```python
from build123d import *

# Parameters (mm, degrees)
SKETCH1_W           = 100
SKETCH1_H           = 40
BOSS_EXTRUDE1_DEPTH = 5
BOSS_EXTRUDE2_DEPTH = 5
SKETCH4_W           = 40
SKETCH4_H           = 12
BOSS_EXTRUDE3_DEPTH = 20
CUT_EXTRUDE2_DEPTH  = 70
BOSS_EXTRUDE5_DEPTH = 100
SKETCH12_R          = 1.4
CUT_EXTRUDE3_DEPTH  = 10
CUT_EXTRUDE4_DEPTH  = 30
BOSS_EXTRUDE6_DEPTH = 25
CUT_EXTRUDE5_DEPTH  = 30
BOSS_EXTRUDE7_DEPTH = 25
FILLET1_R           = 5


with BuildPart() as part:
    # Sketch1 → Boss-Extrude1 (new body)
    with BuildSketch(Plane(origin=(0, 0, 0), x_dir=(1, 0, 0), z_dir=(0, 1, 0))):
        Rectangle(SKETCH1_W, SKETCH1_H)
    extrude(amount=BOSS_EXTRUDE1_DEPTH)

    # Sketch3 → Boss-Extrude2 (add)
    with BuildSketch(Plane(origin=(0, 5, 0), x_dir=(1, 0, 0), z_dir=(0, 1, 0))):
        Polygon((0, 20), (-20, 20), (-20, -20), (20, -20), (20, 20), align=None)
    extrude(amount=BOSS_EXTRUDE2_DEPTH)

    # Sketch4 → Boss-Extrude3 (add)
    with BuildSketch(Plane(origin=(0, 10, 0), x_dir=(1, 0, 0), z_dir=(0, 1, 0))):
        with Locations((0, 14)):
            Rectangle(SKETCH4_W, SKETCH4_H)
        with Locations((0, -14)):
            Rectangle(SKETCH4_W, SKETCH4_H)
    extrude(amount=BOSS_EXTRUDE3_DEPTH)

    # Sketch10 → Cut-Extrude2 (cut)
    with BuildSketch(Plane(origin=(20, 0, 0), x_dir=(0, 0, -1), z_dir=(1, 0, 0))):
        Polygon((-8, 10), (-15, 10), (-15, 15), (-8, 25), align=None)
        Polygon((8, 10), (15, 10), (15, 14.5), (8, 25), align=None)
    extrude(amount=-CUT_EXTRUDE2_DEPTH, mode=Mode.SUBTRACT)

    # Sketch11 → Boss-Extrude5 (add)
    with BuildSketch(Plane.ZY.offset(50)):
        Polygon((20, 0), (-20, -4.911382436), (-20, 0), align=None)
    extrude(amount=-BOSS_EXTRUDE5_DEPTH)

    # Sketch12 → Cut-Extrude3 (cut)
    with BuildSketch(Plane(origin=(0, -2.419218956, 0.297042737), x_dir=(1, 0, 0), z_dir=(0, -0.992546151641323, 0.121869343405141))):
        with Locations(Location((-22.5, 0, 0), (0, 0, 270))):
            Circle(SKETCH12_R)
        with Locations(Location((22.5, 0, 0), (0, 0, 270))):
            Circle(SKETCH12_R)
    extrude(amount=-CUT_EXTRUDE3_DEPTH, mode=Mode.SUBTRACT)

    # Sketch16 → Cut-Extrude4 (cut)
    with BuildSketch(Plane.ZY.offset(50)):
        Polygon((-2.653640591, 5), (1.346359409, 5), (-2.653640591, 4.508861756), align=None)
    extrude(amount=-CUT_EXTRUDE4_DEPTH, mode=Mode.SUBTRACT)

    # Sketch17 → Boss-Extrude6 (add)
    with BuildSketch(Plane.ZY.offset(50)):
        Polygon((-2.653640591, 5), (-2.653640591, 4.508861756), (1.346359409, 5), align=None)
    extrude(amount=-BOSS_EXTRUDE6_DEPTH)

    # Sketch18 → Cut-Extrude5 (cut)
    with BuildSketch(Plane(origin=(50, 0, 0), x_dir=(0, 0, -1), z_dir=(1, 0, 0))):
        Polygon((2.679400207, 5), (-1.320599793, 5), (2.679400207, 4.508861756), align=None)
    extrude(amount=-CUT_EXTRUDE5_DEPTH, mode=Mode.SUBTRACT)

    # Sketch19 → Boss-Extrude7 (add)
    with BuildSketch(Plane(origin=(50, 0, 0), x_dir=(0, 0, -1), z_dir=(1, 0, 0))):
        Polygon((2.679400207, 4.508861756), (2.679400207, 5), (-1.320599793, 5), align=None)
    extrude(amount=-BOSS_EXTRUDE7_DEPTH)

    # Fillet1
    fillet1_edges = [part.edges().sort_by_distance(p)[0] for p in [
        (50, 0.044308782, -20),
        (50, 2.5, 20),
        (-50, 2.5, 20),
        (-50, 0.044308782, -20),
    ]]
    fillet(fillet1_edges, radius=FILLET1_R)


solid = part.part
```
Geometry: final body of the model. Coordinates: model frame, mm. A direction names the side the tool comes from. Coordinates: 2 decimals unless noted, no trailing zeros. Order: outer loops, then holes, each group sorted by start corner. A loop starts at its lowest first (then second) coordinate and runs counter-clockwise, first axis right, second up. Notation, with made-up numbers: (-30, 57.25) - (-14, 57.25) arc R14 cw to (-14, 64.25) - close; hole circle Ø8 at (60, 67.5). An arc over 180 degrees is marked (long way). Write each question's results on one line, items separated by ' | '.
1) Section B-B, the plane y = 18.5. Return loops of the section in (x, z).
Results list:
outline: (-20, -20) - (20, -20) - (20, -12.33) - (-20, -12.33) - close; (-20, 12.55) - (20, 12.55) - (20, 20) - (-20, 20) - close
2) Pin query (flat end, axial travel): pin 1 (20.5 mm diameter, centred on y = 18.5, z = 6.5, fed in from +X); pin 2 (24 mm diameter, centred on x = -36, z = 0, fed in from +Y); pin 3 (4 mm diameter, centred on x = 1, z = -15.5, fed in from -Y). Return the tip coordinate at first contact, or that it passes through.
Results list:
pin 1: x = 20 | pin 2: y = 5 | pin 3: y = -4.6
3) Section C-C, the plane z = -16.5. Return loops of the section in (x, y), plus the area to 3 significant figures.
Results list:
outline: (-49.77, -4.48) - (49.77, -4.48) - (49.77, 5) - (20, 5) - (20, 30) - (-20, 30) - (-20, 5) - (-49.77, 5) - close | area: 1,940 mm^2
4) Set-up query: faces 1 (the flat face through (35, 5, 0)), 2 (the flat face through (0.28, 19.676, -11.549)), 3 (the flat face through (0, 30, 14)), 4 (the flat face through (0, 27, 8)). Return all of +Z, -Z, +X, -X, +Y, -Y with unobstructed straight access to the full face (end or side cutting, diameter ignored); none if empty.
Results list:
face 1: +Z, -Z, +X, +Y | face 2: +X, -X | face 3: +Z, -Z, +X, -X, +Y | face 4: +X, -X, +Y
5) Section A-A, the plane x = -12. Return loops of the section in (y, z).
Results list:
outline: (-4.91, -20) - (30, -20) - (30, -8) - (25, -8) - (14.5, -15) - (10, -15) - (10, 15) - (15, 15) - (25, 8) - (30, 8) - (30, 20) - (0, 20) - close
6) Pull-direction query (X, two-part tool) for faces 5 (the cylindrical face through (21.133, 1.16, 0.163)), 6 (the flat face through (-50, 1, 0)), 7 (the flat face through (0, 30, -14)); classes: pulls with the +X half, pulls with the -X half, needs draft (parallel to the pull), parting line crosses it, or undercut.
Results list:
face 5: undercut | face 6: pulls with the -X half | face 7: needs draft
7) Line query: line 1 (Y direction, x = 41, z = 15); line 2 (Z direction, x = -19.5, y = 21.5); line 3 (X direction, y = 22, z = -11.5). Output: solid intervals per line, ascending. Write a range as from..to.
Results list:
line 1: -0.61..5 | line 2: -20..-10.33, 10.45..20 | line 3: -20..20
8) Section D-D, the plane z = 0. State how many separate pieces and enclosed holes the cut face has, plus the area to 3 significant figures.
Results list:
separate pieces: 3 | enclosed holes: 0 | area: 904 mm^2
